```python
from build123d import *

# Parameters (mm, degrees)
SKETCH_1_W          = 88
SKETCH_1_H          = 88
EXTRUDE_1_DEPTH     = 9.5
SKETCH_2_W          = 88
SKETCH_2_H          = 9.5
EXTRUDE_2_DEPTH     = 88
EXTRUDE_3_DEPTH     = 4.5
SKETCH_4_R          = 4.75
CUT_EXTRUDE_1_DEPTH = 126.866000175


with BuildPart() as part:
    # 草图1 → 凸台-拉伸1 (new body)
    with BuildSketch(Plane.XY):
        Rectangle(SKETCH_1_W, SKETCH_1_H)
    extrude(amount=EXTRUDE_1_DEPTH)

    # 草图2 → 凸台-拉伸2 (add)
    with BuildSketch(Plane(origin=(0, 0, 0), x_dir=(-1, 0, 0), z_dir=(0, 0, -1))):
        with Locations((0, -39.25)):
            Rectangle(SKETCH_2_W, SKETCH_2_H)
    extrude(amount=-EXTRUDE_2_DEPTH)

    # 草图3 → 凸台-拉伸3 (add)
    with BuildSketch(Plane.ZY.offset(44)):
        Polygon((9.5, 44), (88, -34.5), (9.5, -34.5), align=None)
    extrude_3 = extrude(amount=-EXTRUDE_3_DEPTH)

    # 镜向1: 凸台-拉伸3 across plane
    add(extrude_3.mirror(Plane(origin=(0, 0, 0), x_dir=(0, 0, 1), z_dir=(1, 0, 0))))

    # 草图4 → 切除-拉伸1 (cut, through all)
    with BuildSketch(Plane(origin=(0, -34.5, 0), x_dir=(1, 0, 0), z_dir=(0, 1, 0))):
        with Locations(Location((22.5, -63.5, 0), (0, 0, 270))):
            Circle(SKETCH_4_R)
        with Locations(Location((-22.5, -63.5, 0), (0, 0, 90))):
            Circle(SKETCH_4_R)
        with BuildLine():
            Line((17.75, -37.7), (17.75, -22.2))
            ThreePointArc((17.75, -22.2), (22.5, -17.45), (27.25, -22.2))
            Line((27.25, -22.2), (27.25, -37.7))
            ThreePointArc((27.25, -37.7), (22.5, -42.45), (17.75, -37.7))
        make_face()
        with BuildLine():
            Line((-17.75, -37.7), (-17.75, -22.2))
            ThreePointArc((-17.75, -22.2), (-22.5, -17.45), (-27.25, -22.2))
            Line((-27.25, -22.2), (-27.25, -37.7))
            ThreePointArc((-27.25, -37.7), (-22.5, -42.45), (-17.75, -37.7))
        make_face()
    cut_extrude_1 = extrude(amount=-CUT_EXTRUDE_1_DEPTH, mode=Mode.SUBTRACT)

    # 镜向2: 切除-拉伸1 across plane
    add(cut_extrude_1.mirror(Plane(origin=(0, -22, 22), x_dir=(0, 0.7071067811865476, 0.7071067811865476), z_dir=(0, -0.7071067811865477, 0.7071067811865475))), mode=Mode.SUBTRACT)


solid = part.part
```
Here's how the part is built. I have some questions about the finished solid (model axes, mm). A direction names the side the tool comes from. Coordinates: 2 decimals unless noted, no trailing zeros. Loops run counter-clockwise (first coordinate to the right, second up) from the corner with the lowest first, then second, coordinate; pieces in that order, holes last. Notation, with made-up numbers: M -28.5,52.5 L -16.5,52.5 A20 ccw -16.5,81.5 Z; hole C 22.5,-19 d5. An arc over 180 degrees is marked long. One line per item, written item: value.
1. Thinking about a two-plate mould opening in Y: for faces 4 (the flat face through (41.8, 5.3, 48.2)), 5 (the flat face through (-1, -44, 43)), 6 (the cylindrical face through (-22.4, -26.55, 4.82)), 7 (the cylindrical face through (25.71, -39.18, 60)), which applies, +Y half, -Y half, draft (parallel to the pull), parting line (faces both ways), or undercut?
Geometry says:
face 4: +Y half
face 5: -Y half
face 6: undercut
face 7: draft
2. Please list where these lines run through material, in increasing order: probe 1 along X at (y, z) = (-36, 63); probe 2 along Y at (x, z) = (22, 3); probe 3 along Z at (x, y) = (-22.5, -40.75).
Geometry says:
probe 1: x = -44 to -27.22, -17.78 to 17.78, 27.22 to 44
probe 2: y = -44 to -26.52, -1.58 to 14.78, 24.22 to 44
probe 3: z = 0 to 17.45, 42.45 to 58.75, 68.25 to 88
3. Imagine slicing it at A-A (y = 19.5). List the corners of the cut face in (x, z) for me.
Geometry says:
outline: M -44,0 L -27.25,0 L -27.25,9.5 L -39.5,9.5 L -39.5,34 L -44,34 Z; M -17.75,0 L 17.75,0 L 17.75,9.5 L -17.75,9.5 Z; M 27.25,0 L 44,0 L 44,34 L 39.5,34 L 39.5,9.5 L 27.25,9.5 Z
4. Imagine slicing it at B-B (z = 34). List the corners of the cut face in (x, y) for me, and give its area (3 significant figures).
Geometry says:
outline: M -44,-44 L -27.25,-44 L -27.25,-34.5 L -39.5,-34.5 L -39.5,19.5 L -44,19.5 Z; M -17.75,-44 L 17.75,-44 L 17.75,-34.5 L -17.75,-34.5 Z; M 27.25,-44 L 44,-44 L 44,19.5 L 39.5,19.5 L 39.5,-34.5 L 27.25,-34.5 Z
area: 1,140 mm2
5. Imagine slicing it at C-C (x = 22.5). List the corners of the cut face in (y, z) for me.
Geometry says:
outline: M -44,0 L -26.55,0 L -26.55,9.5 L -34.5,9.5 L -34.5,17.45 L -44,17.45 Z; M -44,42.45 L -34.5,42.45 L -34.5,58.75 L -44,58.75 Z; M -44,68.25 L -34.5,68.25 L -34.5,88 L -44,88 Z; M -1.55,0 L 14.75,0 L 14.75,9.5 L -1.55,9.5 Z; M 24.25,0 L 44,0 L 44,9.5 L 24.25,9.5 Z
6. Imagine slicing it at D-D (y = 35). List the corners of the cut face in (x, z) for me, and give its area (3 significant figures).
Geometry says:
outline: M -44,0 L 44,0 L 44,18.5 L 39.5,18.5 L 39.5,9.5 L -39.5,9.5 L -39.5,18.5 L -44,18.5 Z
area: 917 mm2
7. Will these pins go through, and if not, where does the flat tip stop? pin 1 Ø5 at (y, z) = (-10, 65) entering from -X; pin 2 Ø1 at (x, z) = (30.5, 50.5) entering from +Y; pin 3 Ø5 at (x, y) = (-33, 23.5) entering from +Z.
Geometry says:
pin 1: stops at x = -44
pin 2: stops at y = -34.5
pin 3: stops at z = 9.5
8. On a 3-axis mill with a long thin cutter (end or side, diameter ignored), from which of +Z, -Z, +X, -X, +Y, -Y can I reach the whole of each face in a straight line? I mean faces 1 (the flat face through (27.25, -39, 30)), 2 (the flat face through (-17.75, -14, 5)), 3 (the flat face through (1, -34.5, 48)). Say none if no direction works.
Geometry says:
face 1: +Y, -Y
face 2: +Z, -Z
face 3: +Z, +Y
